Input: part model. Units: mm. Frame: model coordinates. A direction names the side the tool comes from. Round coordinates to 2 decimals unless told otherwise and drop trailing zeros. Loops run counter-clockwise (first coordinate to the right, second up) from the corner with the lowest first, then second, coordinate; pieces in that order, holes last.
1) Section A-A, the plane y = 18.5. Return loops of the section in (x, z).
2) Ray query, line 1 along Z through (x, y) = (1, 0); line 2 along Y through (x, z) = (0.75, 24); line 3 along Z through (x, y) = (-4.25, 0). Return the intervals inside material, ascending.
3) First-contact query: pin 1 (22 mm diameter, centred on y = -27, z = 0, fed in from -X); pin 2 (5 mm diameter, centred on x = -2, y = -21, fed in from -Z); pin 3 (4.5 mm diameter, centred on x = -3, y = 50, fed in from -Z); pin 4 (1 mm diameter, centred on x = 5, z = -22.5, fed in from -Y). Flat tips, straight axial feed; report the tip coordinate or a pass-through.
4) Section D-D, the plane x = 5. State how many separate pieces and enclosed holes the cut face has, and give its area (3 significant figures).
5) Section B-B, the plane z = -6.5. Return loops of the section in (x, y), and give its area (3 significant figures).
6) Section C-C, the plane y = 41.5. Return loops of the section in (x, z).
7) Access query for faces 1 (the face through (-0.111, 3.103, -30.3)), 2 (the face through (0.11, 48.33, -21.8)). Directions: +Z, -Z, +X, -X, +Y, -Y. A direction counts if a zero-diameter tool reaches every point of the face in a straight line with its end or side. Return the directions, or none.
8) Draft query along Y for faces 3 (the face through (1.185, 51.219, 22.686)), 4 (the face through (0.111, 15.213, -30.891)), 5 (the face through (0, 22, -30.5)). Return one class per face: pulls with the +Y half, pulls with the -Y half, needs draft (parallel to the pull), parting line crosses it, or undercut.
from build123d import *
from build123d.topology import SkipClean

# Parameters (mm, degrees)
BOSS_EXTRUDE1_DEPTH     = 8
CUT_EXTRUDE1_DEPTH      = 78.453287602
CUT_EXTRUDE1_DEPTH_BACK = 70.453287602
CUT_EXTRUDE1_START      = -8
SKETCH9_R               = 5
CUT_EXTRUDE2_DEPTH      = 70.453287602
CUT_EXTRUDE2_DEPTH_BACK = 70.453287602
CUT_EXTRUDE3_DEPTH      = 70.453287602
CUT_EXTRUDE3_DEPTH_BACK = 70.453287602
SKETCH11_R              = 18.5
CUT_EXTRUDE4_DEPTH      = 70.453287602
CUT_EXTRUDE4_DEPTH_BACK = 70.453287602
SKETCH12_W              = 5.7
SKETCH12_H              = 2.4
CUT_EXTRUDE5_START      = 27.875085
CUT_EXTRUDE5_DEPTH      = 6
MOVE_START              = -8
MOVE_FACE1_OUTLINE_W    = 5.7
MOVE_FACE1_OUTLINE_H    = 2.4
MOVE_FACE1_OUTLINE_R    = 18.5
MOVE_FACE1_DEPTH        = 0.1
MOVE_START_2            = 7.9
MOVE_FACE1_2_OUTLINE_W  = 5.7
MOVE_FACE1_2_OUTLINE_H  = 2.4
MOVE_FACE1_2_OUTLINE_R  = 18.5
MOVE_FACE1_2_DEPTH      = 0.1


# Read off the part's stored shape, not the designer's step: Move Face1
with BuildPart() as part:
    # Sketch2 → Boss-Extrude1 (new, symmetric)
    with BuildSketch(Plane.YZ):
        with BuildLine():
            Line((-12.727922061, -32.852837258), (-13.616293225, -31.964466094))
            ThreePointArc((-13.616293225, -31.964466094), (-15.238409969, -30.880602337), (-17.151827131, -30.5))
            Line((-17.151827131, -30.5), (-27, -30.5))
            ThreePointArc((-27, -30.5), (-48.566756826, -21.566756826), (-57.5, 0))
            Line((-57.5, 0), (-57.5, 27.875084803))
            Line((-57.5, 27.875084803), (0, 27.875084803))
            Line((0, 27.875084803), (0, -38.124915197))
            ThreePointArc((0, -38.124915197), (-6.888301783, -36.754746782), (-12.727922061, -32.852837258))
        make_face()
    extrude(amount=BOSS_EXTRUDE1_DEPTH, both=True)

    # Sketch9 → Cut-Extrude1 (cut, two sides: drawn at the far end of the back side and taken through both)
    with BuildSketch(Plane.YZ.offset(CUT_EXTRUDE1_START - CUT_EXTRUDE1_DEPTH_BACK)):
        with Locations((0, 3.875084803)):
            Circle(SKETCH9_R)
        with Locations((0, -20.124915197)):
            Circle(SKETCH9_R)
    extrude(amount=CUT_EXTRUDE1_DEPTH + CUT_EXTRUDE1_DEPTH_BACK, mode=Mode.SUBTRACT)

    # Sketch10 → Cut-Extrude2 (cut, two sides: drawn at the far end of the back side and taken through both)
    with BuildSketch(Plane.YZ.offset(-CUT_EXTRUDE2_DEPTH_BACK)):
        Polygon((2.078460969, 12.275084803), (4.156921938, 15.875084803), (2.078460969, 19.475084803), (-2.078460969, 19.475084803), (-4.156921938, 15.875084803), (-2.078460969, 12.275084803), align=None)
        Polygon((-5.545893683, -31.549584262), (-4.470003116, -27.534306004), (-7.409390808, -24.594918313), (-11.424669066, -25.67080888), (-12.500559632, -29.686087138), (-9.561171941, -32.625474829), align=None)
        Polygon((4.156921938, -32.124915197), (2.078460969, -28.524915197), (-2.078460969, -28.524915197), (-4.156921938, -32.124915197), (-2.078460969, -35.724915197), (2.078460969, -35.724915197), align=None)
        Polygon((12.500559632, -29.686087138), (11.424669066, -25.67080888), (7.409390808, -24.594918313), (4.470003116, -27.534306004), (5.545893683, -31.549584262), (9.561171941, -32.625474829), align=None)
    extrude(amount=CUT_EXTRUDE2_DEPTH + CUT_EXTRUDE2_DEPTH_BACK, mode=Mode.SUBTRACT)

    # Sketch11 → Cut-Extrude3 (cut, two sides: drawn at the far end of the back side and taken through both)
    with BuildSketch(Plane.YZ.offset(-CUT_EXTRUDE3_DEPTH_BACK)):
        with Locations(Location((-27, 0, 0), (0, 0, 270))):
            Circle(SKETCH11_R)
    extrude(amount=CUT_EXTRUDE3_DEPTH + CUT_EXTRUDE3_DEPTH_BACK, mode=Mode.SUBTRACT)

    # Sketch12 → Cut-Extrude4 (cut, two sides: drawn at the far end of the back side and taken through both)
    with BuildSketch(Plane.YZ.offset(-CUT_EXTRUDE4_DEPTH_BACK)):
        with Locations((-50, 24.675084803)):
            Rectangle(SKETCH12_W, SKETCH12_H)
        with Locations((0, 24.675084803)):
            Rectangle(SKETCH12_W, SKETCH12_H)
    extrude(amount=CUT_EXTRUDE4_DEPTH + CUT_EXTRUDE4_DEPTH_BACK, mode=Mode.SUBTRACT)

    # Sketch13 → Cut-Extrude5 (cut)
    with BuildSketch(Plane.XY.offset(CUT_EXTRUDE5_START)):
        Polygon((0, -2.404163056), (2.404163056, 0), (0, 2.404163056), (-2.404163056, 0), align=None)
        Polygon((0, -52.404163056), (2.404163056, -50), (0, -47.595836944), (-2.404163056, -50), align=None)
    extrude(amount=-CUT_EXTRUDE5_DEPTH, mode=Mode.SUBTRACT)

    # Move Face1 outline → Move Face1 (cut)
    with BuildSketch(Plane.YZ.offset(MOVE_START)):
        with BuildLine():
            Line((-2.85, 25.875084803), (0, 25.875084803))
            Line((0, 25.875084803), (0, 27.875084803))
            Line((0, 27.875084803), (-57.5, 27.875084803))
            Line((-57.5, 27.875084803), (-57.5, 0))
            ThreePointArc((-57.5, 0), (-48.566756826, -21.566756826), (-27, -30.5))
            Line((-27, -30.5), (-17.151827131, -30.5))
            ThreePointArc((-17.151827131, -30.5), (-15.238409969, -30.880602337), (-13.616293225, -31.964466094))
            Line((-13.616293225, -31.964466094), (-12.727922061, -32.852837258))
            ThreePointArc((-12.727922061, -32.852837258), (-6.888301783, -36.754746782), (0, -38.124915197))
            Line((0, -38.124915197), (0, -35.724915197))
            Line((0, -35.724915197), (-2.078460969, -35.724915197))
            Line((-2.078460969, -35.724915197), (-4.156921938, -32.124915197))
            Line((-4.156921938, -32.124915197), (-2.078460969, -28.524915197))
            Line((-2.078460969, -28.524915197), (0, -28.524915197))
            Line((0, -28.524915197), (0, -25.124915197))
            ThreePointArc((0, -25.124915197), (-5, -20.124915197), (0, -15.124915197))
            Line((0, -15.124915197), (0, -1.124915197))
            ThreePointArc((0, -1.124915197), (-5, 3.875084803), (0, 8.875084803))
            Line((0, 8.875084803), (0, 12.275084803))
            Line((0, 12.275084803), (-2.078460969, 12.275084803))
            Line((-2.078460969, 12.275084803), (-4.156921938, 15.875084803))
            Line((-4.156921938, 15.875084803), (-2.078460969, 19.475084803))
            Line((-2.078460969, 19.475084803), (0, 19.475084803))
            Line((0, 19.475084803), (0, 23.475084803))
            Line((0, 23.475084803), (-2.85, 23.475084803))
            Line((-2.85, 23.475084803), (-2.85, 25.875084803))
        make_face()
        Polygon((-5.545893683, -31.549584262), (-9.561171941, -32.625474829), (-12.500559632, -29.686087138), (-11.424669066, -25.67080888), (-7.409390808, -24.594918313), (-4.470003116, -27.534306004), align=None, mode=Mode.SUBTRACT)
        with Locations((-50, 24.675084803)):
            Rectangle(MOVE_FACE1_OUTLINE_W, MOVE_FACE1_OUTLINE_H, mode=Mode.SUBTRACT)
        with Locations((-27, 0)):
            Circle(MOVE_FACE1_OUTLINE_R, mode=Mode.SUBTRACT)
    extrude(amount=MOVE_FACE1_DEPTH, mode=Mode.SUBTRACT)

    # Move Face1 2 outline → Move Face1 2 (cut)
    with BuildSketch(Plane.YZ.offset(MOVE_START_2)):
        with BuildLine():
            Line((-2.85, 25.875084803), (0, 25.875084803))
            Line((0, 25.875084803), (0, 27.875084803))
            Line((0, 27.875084803), (-57.5, 27.875084803))
            Line((-57.5, 27.875084803), (-57.5, 0))
            ThreePointArc((-57.5, 0), (-48.566756826, -21.566756826), (-27, -30.5))
            Line((-27, -30.5), (-17.151827131, -30.5))
            ThreePointArc((-17.151827131, -30.5), (-15.238409969, -30.880602337), (-13.616293225, -31.964466094))
            Line((-13.616293225, -31.964466094), (-12.727922061, -32.852837258))
            ThreePointArc((-12.727922061, -32.852837258), (-6.888301783, -36.754746782), (0, -38.124915197))
            Line((0, -38.124915197), (0, -35.724915197))
            Line((0, -35.724915197), (-2.078460969, -35.724915197))
            Line((-2.078460969, -35.724915197), (-4.156921938, -32.124915197))
            Line((-4.156921938, -32.124915197), (-2.078460969, -28.524915197))
            Line((-2.078460969, -28.524915197), (0, -28.524915197))
            Line((0, -28.524915197), (0, -25.124915197))
            ThreePointArc((0, -25.124915197), (-5, -20.124915197), (0, -15.124915197))
            Line((0, -15.124915197), (0, -1.124915197))
            ThreePointArc((0, -1.124915197), (-5, 3.875084803), (0, 8.875084803))
            Line((0, 8.875084803), (0, 12.275084803))
            Line((0, 12.275084803), (-2.078460969, 12.275084803))
            Line((-2.078460969, 12.275084803), (-4.156921938, 15.875084803))
            Line((-4.156921938, 15.875084803), (-2.078460969, 19.475084803))
            Line((-2.078460969, 19.475084803), (0, 19.475084803))
            Line((0, 19.475084803), (0, 23.475084803))
            Line((0, 23.475084803), (-2.85, 23.475084803))
            Line((-2.85, 23.475084803), (-2.85, 25.875084803))
        make_face()
        Polygon((-5.545893683, -31.549584262), (-9.561171941, -32.625474829), (-12.500559632, -29.686087138), (-11.424669066, -25.67080888), (-7.409390808, -24.594918313), (-4.470003116, -27.534306004), align=None, mode=Mode.SUBTRACT)
        with Locations((-50, 24.675084803)):
            Rectangle(MOVE_FACE1_2_OUTLINE_W, MOVE_FACE1_2_OUTLINE_H, mode=Mode.SUBTRACT)
        with Locations((-27, 0)):
            Circle(MOVE_FACE1_2_OUTLINE_R, mode=Mode.SUBTRACT)
    extrude(amount=MOVE_FACE1_2_DEPTH, mode=Mode.SUBTRACT)

    # Mirror1: part across plane


with BuildPart() as part_1:
    with SkipClean():  # the faces are left unmerged after this step: merging them gives an invalid solid
        add(part.part)
        add(part.part.mirror(Plane(origin=(0, 0, 0), x_dir=(0, 0, 1), z_dir=(0, -1, 0))))


solid = part_1.part
Final values:
1. outline: (-7.9, -30.5) - (7.9, -30.5) - (7.9, -16.43) - (-7.9, -16.43) - close; (-7.9, 16.43) - (7.9, 16.43) - (7.9, 27.88) - (-7.9, 27.88) - close
2. line 1: z = -38.12 to -35.72, -28.52 to -25.12, -15.12 to -1.12, 8.88 to 12.28, 19.48 to 21.88
2. line 2: y = -57.5 to -52.85, -47.15 to -2.85, 2.85 to 47.15, 52.85 to 57.5
2. line 3: z = -38.12 to -35.72, -28.52 to -25.12, -15.12 to -1.12, 8.88 to 12.28, 19.48 to 23.48, 25.88 to 27.88
3. pin 1: passes through
3. pin 2: stops at z = -30.5
3. pin 3: stops at z = -22.35
3. pin 4: stops at y = -48.12
4. separate pieces: 1
4. enclosed holes: 11
4. area: 3,940 mm2
5. outline: (-7.9, -56.8) - (7.9, -56.8) - (7.9, -44.32) - (-7.9, -44.32) - close; (-7.9, -9.68) - (7.9, -9.68) - (7.9, 9.68) - (-7.9, 9.68) - close; (-7.9, 44.32) - (7.9, 44.32) - (7.9, 56.8) - (-7.9, 56.8) - close
5. area: 700 mm2
6. outline: (-7.9, -26.83) - (7.9, -26.83) - (7.9, -11.49) - (-7.9, -11.49) - close; (-7.9, 11.49) - (7.9, 11.49) - (7.9, 27.88) - (-7.9, 27.88) - close
7. face 1: +X, -X
7. face 2: -Z, +X, -X, +Y
8. face 3: undercut
8. face 4: pulls with the +Y half
8. face 5: needs draft
